Geometry: final body of the model. Coordinates: model frame, mm. A direction names the side the tool comes from. Give positions to 0.01 mm unless a question says otherwise; leave off trailing zeros. Order: outer loops, then holes, each group sorted by start corner. A loop starts at its lowest first (then second) coordinate and runs counter-clockwise, first axis right, second up. Notation, with made-up numbers: M -14,-14.75 L 9,-14.75 A12 ccw 9,6.25 Z; hole C 60,23 d11. An arc over 180 degrees is marked long. Write item = value, one per line. Start each with the question number.
from build123d import *

# Parameters (mm, degrees)
SKICA2_R                 = 1.75
SKICA2_W                 = 18.35
SKICA2_H                 = 23.35
P_IDAT_VYSUNUT_M1_DEPTH  = 6
SKICA2_3_R               = 1.5
P_IDAT_VYSUNUT_M2_DEPTH  = 4
SKICA4_W                 = 18.35
SKICA4_H                 = 3.325
ODEBRAT_VYSUNUT_M2_DEPTH = 29.91366459
ODEBRAT_START            = -1
SKICA5_R                 = 2.5
SKICA5_R_2               = 1.5
ODEBRAT_VYSUNUT_M3_DEPTH = 1
ZKOSEN_1_SIZE            = 0.6
ZAOBLIT1_R               = 2
ZAOBLIT2_R               = 1


with BuildPart() as part:
    # Skica2 → P_idat vysunut_m1 (new body)
    with BuildSketch(Plane.XY):
        with BuildLine():
            Line((-20, 13), (-20, -15))
            Line((-20, -15), (20, -15))
            Line((20, -15), (20, 13))
            ThreePointArc((20, 13), (19.847759065, 13.765366865), (19.414213562, 14.414213562))
            Line((19.414213562, 14.414213562), (13.828427125, 20))
            Line((13.828427125, 20), (-13.828427125, 20))
            Line((-13.828427125, 20), (-19.414213562, 14.414213562))
            ThreePointArc((-19.414213562, 14.414213562), (-19.847759065, 13.765366865), (-20, 13))
        make_face()
        with Locations((-15, 0)):
            Circle(SKICA2_R, mode=Mode.SUBTRACT)
        with Locations((15, 0)):
            Circle(SKICA2_R, mode=Mode.SUBTRACT)
        Rectangle(SKICA2_W, SKICA2_H, mode=Mode.SUBTRACT)
    extrude(amount=-P_IDAT_VYSUNUT_M1_DEPTH)

    # Skica2_3 → P_idat vysunut_m2 (add)
    with BuildSketch(Plane.XY):
        with Locations((-15, -10)):
            Circle(SKICA2_3_R)
        with Locations((15, -10)):
            Circle(SKICA2_3_R)
        with Locations((15, 10)):
            Circle(SKICA2_3_R)
        with Locations((-15, 10)):
            Circle(SKICA2_3_R)
    extrude(amount=P_IDAT_VYSUNUT_M2_DEPTH)

    # Skica4 → Odebrat vysunut_m2 (cut, through all)
    with BuildSketch(Plane.XY):
        with Locations((0, -13.3375)):
            Rectangle(SKICA4_W, SKICA4_H)
    extrude(amount=-ODEBRAT_VYSUNUT_M2_DEPTH, mode=Mode.SUBTRACT)

    # Skica5 → Odebrat vysunut_m3 (cut)
    # profile 1 of 4: a face of its own
    with BuildSketch(Plane.XY.offset(ODEBRAT_START)):
        with Locations((-15, 10)):
            Circle(SKICA5_R)
        with Locations((-15, 10)):
            Circle(SKICA5_R_2, mode=Mode.SUBTRACT)
    # profile 2 of 4: a face of its own
    with BuildSketch(Plane.XY.offset(ODEBRAT_START)):
        with Locations((-15, -10)):
            Circle(SKICA5_R)
        with Locations((-15, -10)):
            Circle(SKICA5_R_2, mode=Mode.SUBTRACT)
    # profile 3 of 4: a face of its own
    with BuildSketch(Plane.XY.offset(ODEBRAT_START)):
        with Locations((15, -10)):
            Circle(SKICA5_R)
        with Locations((15, -10)):
            Circle(SKICA5_R_2, mode=Mode.SUBTRACT)
    # profile 4 of 4: a face of its own
    with BuildSketch(Plane.XY.offset(ODEBRAT_START)):
        with Locations((15, 10)):
            Circle(SKICA5_R)
        with Locations((15, 10)):
            Circle(SKICA5_R_2, mode=Mode.SUBTRACT)
    extrude(amount=ODEBRAT_VYSUNUT_M3_DEPTH, mode=Mode.SUBTRACT)

    # Zkosen_1
    zkosen_1_edges = [part.edges().sort_by_distance(p)[0] for p in [
        (-16.5, 10, 4),
        (13.5, 10, 4),
        (13.5, -10, 4),
        (-16.5, -10, 4),
    ]]
    chamfer(zkosen_1_edges, length=ZKOSEN_1_SIZE)

    # Zaoblit1
    zaoblit1_edges = [part.edges().sort_by_distance(p)[0] for p in [
        (-13.828427125, 20, -3),
        (13.828427125, 20, -3),
        (20, -15, -3),
        (-20, -15, -3),
        (9.175, -15, -3),
        (-9.175, -15, -3),
    ]]
    fillet(zaoblit1_edges, radius=ZAOBLIT1_R)

    # Zaoblit2
    zaoblit2_edges = [part.edges().sort_by_distance(p)[0] for p in [
        (-9.175, 11.675, -3),
        (9.175, 11.675, -3),
    ]]
    fillet(zaoblit2_edges, radius=ZAOBLIT2_R)


solid = part.part
1) Cut plane A-A (y = -6). Return loops of the section in (x, z) (3 decimals), plus the area to 3 significant figures.
2) Ray query, L1, parallel to X at y = -3, z = -5.5 (3 decimals); L2, parallel to Y at x = 15, z = -0.4; L3, parallel to Z at x = 10, y = 13.5. Return the intervals inside material, ascending.
3) Cut plane B-B (z = -3.5). Return loops of the section in (x, y) (3 decimals), plus the area to 3 significant figures.
4) Cut plane D-D (y = -10). Return loops of the section in (x, z) (3 decimals).
5) Cut plane C-C (x = 15). Return loops of the section in (y, z).
6) Access query for faces 5 (the cylindrical face through (-17, 8.5, -0.5)), 6 (the flat face through (20, 0, -3)), 7 (the flat face through (9.175, -1, -3)). Directions: +Z, -Z, +X, -X, +Y, -Y. A direction counts if a zero-diameter tool reaches every point of the face in a straight line with its end or side. Return the directions, or none.
7) Draft query along Y for faces 1 (the cylindrical face through (-19.84, 13.78, -2.96)), 2 (the flat face through (-15, 8, -1)), 3 (the cylindrical face through (13, -11.5, -0.5)), 4 (the flat face through (-9.175, -1, -3)). Return one class per face: pulls with the +Y half, pulls with the -Y half, needs draft (parallel to the pull), parting line crosses it, or undercut.
8) Pin query (flat end, axial travel): pin 1 Ø4 at (x, y) = (-15, 0) entering from +Z; pin 2 Ø2 at (y, z) = (14.5, 0) entering from +X; pin 3 Ø3 at (x, z) = (5.5, -2.5) entering from -Y (3 decimals). Return the tip coordinate at first contact, or that it passes through.
Reply:
q1.outline = M -20,-6 L -9.175,-6 L -9.175,0 L -20,0 Z; M 9.175,-6 L 20,-6 L 20,0 L 9.175,0 Z
q1.area = 130 mm²
q2.L1 = -20 to -9.175, 9.175 to 20
q2.L2 = -15 to -12.5, -11.5 to -8.5, -7.5 to -1.75, 1.75 to 7.5, 8.5 to 11.5, 12.5 to 18.83
q2.L3 = -6 to 0
q3.outline = M -20,-13 A2 ccw -18,-15 L -11.175,-15 A2 ccw -9.175,-13 L -9.175,10.675 A1 cw -8.175,11.675 L 8.175,11.675 A1 cw 9.175,10.675 L 9.175,-13 A2 ccw 11.175,-15 L 18,-15 A2 ccw 20,-13 L 20,13 A2 ccw 19.414,14.414 L 14.414,19.414 A2 ccw 13,20 L -13,20 A2 ccw -14.414,19.414 L -19.414,14.414 A2 ccw -20,13 Z; hole C -15,0 d3.5; hole C 15,0 d3.5
q3.area = 850 mm²
q4.outline = M -20,-6 L -9.175,-6 L -9.175,0 L -12.5,0 L -12.5,-1 L -13.5,-1 L -13.5,3.4 L -14.1,4 L -15.9,4 L -16.5,3.4 L -16.5,-1 L -17.5,-1 L -17.5,0 L -20,0 Z; M 9.175,-6 L 20,-6 L 20,0 L 17.5,0 L 17.5,-1 L 16.5,-1 L 16.5,3.4 L 15.9,4 L 14.1,4 L 13.5,3.4 L 13.5,-1 L 12.5,-1 L 12.5,0 L 9.175,0 Z
q5.outline = M -15,-6 L -1.75,-6 L -1.75,0 L -7.5,0 L -7.5,-1 L -8.5,-1 L -8.5,3.4 L -9.1,4 L -10.9,4 L -11.5,3.4 L -11.5,-1 L -12.5,-1 L -12.5,0 L -15,0 Z; M 1.75,-6 L 18.83,-6 L 18.83,0 L 12.5,0 L 12.5,-1 L 11.5,-1 L 11.5,3.4 L 10.9,4 L 9.1,4 L 8.5,3.4 L 8.5,-1 L 7.5,-1 L 7.5,0 L 1.75,0 Z
q6.face_5 = +Z
q6.face_6 = +Z, -Z, +X, +Y, -Y
q6.face_7 = +Z, -Z, -Y
q7.face_1 = pulls with the +Y half
q7.face_2 = undercut
q7.face_3 = undercut
q7.face_4 = needs draft
q8.pin_1 = 0
q8.pin_2 = 19.94
q8.pin_3 = 11.675
